from build123d import *

# Parameters (mm, degrees)
SKETCH1_W           = 7.5
SKETCH1_H           = 7.5
BOSS_EXTRUDE1_DEPTH = 40
SKETCH2_W           = 24
SKETCH2_H           = 20
BOSS_EXTRUDE2_DEPTH = 40
SKETCH4_R           = 3.75
CUT_EXTRUDE1_DEPTH  = 20
SKETCH3_R           = 3.25
CUT_EXTRUDE2_DEPTH  = 40


with BuildPart() as part:
    # Sketch1 → Boss-Extrude1 (new body)
    with BuildSketch(Plane(origin=(0, 0, 0), x_dir=(0, 0, -1), z_dir=(1, 0, 0))):
        Rectangle(SKETCH1_W, SKETCH1_H)
    extrude(amount=BOSS_EXTRUDE1_DEPTH)

    # Sketch2 → Boss-Extrude2 (add)
    with BuildSketch(Plane.ZY):
        Rectangle(SKETCH2_W, SKETCH2_H)
    extrude(amount=BOSS_EXTRUDE2_DEPTH)

    # Sketch4 → Cut-Extrude1 (cut)
    with BuildSketch(Plane(origin=(0, 10, 0), x_dir=(1, 0, 0), z_dir=(0, 1, 0))):
        with Locations((-30, 0)):
            Circle(SKETCH4_R)
    extrude(amount=-CUT_EXTRUDE1_DEPTH, mode=Mode.SUBTRACT)

    # Sketch3 → Cut-Extrude2 (cut)
    with BuildSketch(Plane(origin=(40, 0, 0), x_dir=(0, 0, -1), z_dir=(1, 0, 0))):
        Circle(SKETCH3_R)
    extrude(amount=-CUT_EXTRUDE2_DEPTH, mode=Mode.SUBTRACT)


solid = part.part
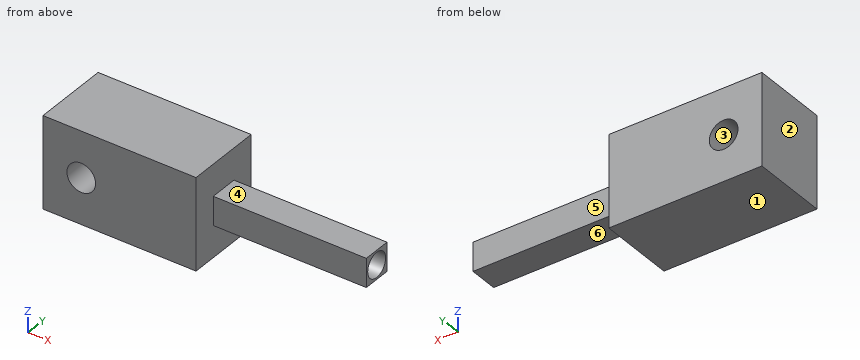
Could you check a few things on this model? Use its own coordinates, in mm. Face numbers are marked on the shaded views. A direction names the side the tool comes from. Round coordinates to 2 decimals unless told otherwise and drop trailing zeros. Write each loop counter-clockwise with the first axis right and the second up, starting at its lowest first coordinate (ties: lowest second). Pieces come first, ordered by that corner, then holes. Notation, with made-up numbers: (65.25, -11) -> (85.25, -11) arc R22 cw to (85.25, 3) -> close; hole circle Ø8 at (-26, 49). An arc over 180 degrees is marked (long way). Use a Markdown table: item, result.
1. We'd pull the mould along Z, two halves only. Please class the marked faces 1, 2 and 3: +Z half, -Z half, draft (parallel to the pull), parting line (faces both ways), or undercut.
Answer key:
| item | result |
|---|---|
| face 1 | -Z half |
| face 2 | draft |
| face 3 | undercut |
2. If we section it at B-B (z = 0): List the corners of the cut face in (x, y) for me.
Answer key:
| item | result |
|---|---|
| outline | (-40, -10) -> (-33.75, -10) -> (-33.75, 10) -> (-40, 10) -> close; (-26.25, -10) -> (0, -10) -> (0, -3.75) -> (40, -3.75) -> (40, -3.25) -> (0, -3.25) -> (0, 3.25) -> (40, 3.25) -> (40, 3.75) -> (0, 3.75) -> (0, 10) -> (-26.25, 10) -> close |
3. Please list where these lines run through material, in increasing order: probe 1 along Y at (x, z) = (14, 0); probe 2 along Z at (x, y) = (-30, 3.75); probe 3 along X at (y, z) = (1, -2.75).
Answer key:
| item | result |
|---|---|
| probe 1 | y = -3.75 to -3.25, 3.25 to 3.75 |
| probe 2 | z = -12 to -3.75, 3.75 to 12 |
| probe 3 | x = -40 to -32.55, -27.45 to 0 |
4. If we section it at C-C (y = 0): List the corners of the cut face in (x, z) for me, then the cut area to 3 significant figures.
Answer key:
| item | result |
|---|---|
| outline | (-40, -12) -> (0, -12) -> (0, -3.75) -> (40, -3.75) -> (40, -3.25) -> (0, -3.25) -> (0, 3.25) -> (40, 3.25) -> (40, 3.75) -> (0, 3.75) -> (0, 12) -> (-40, 12) -> close; hole circle Ø7.5 at (-30, 0) |
| area | 956 mm^2 |
5. If we section it at D-D (x = 17): List the corners of the cut face in (y, z) for me.
Answer key:
| item | result |
|---|---|
| outline | (-3.75, -3.75) -> (3.75, -3.75) -> (3.75, 3.75) -> (-3.75, 3.75) -> close; hole circle Ø6.5 at (0, 0) |
6. If we section it at A-A (x = -27): List the corners of the cut face in (y, z) for me.
Answer key:
| item | result |
|---|---|
| outline | (-10, -12) -> (10, -12) -> (10, -2.25) -> (-10, -2.25) -> close; (-10, 2.25) -> (10, 2.25) -> (10, 12) -> (-10, 12) -> close |
7. For pin 1 Ø4 at (x, z) = (15.5, -1.5) entering from -Y; pin 2 Ø2 at (x, y) = (21, 0.5) entering from -Z; pin 3 Ø2 at (x, y) = (15, 2) entering from +Z; pin 4 Ø10 at (y, z) = (-5, 3.5) entering from +X, each with a flat end and sliding along its axis, tell me the tip position at first contact or that it passes through.
Answer key:
| item | result |
|---|---|
| pin 1 | stops at y = -3.75 |
| pin 2 | stops at z = -3.75 |
| pin 3 | stops at z = 3.75 |
| pin 4 | stops at x = 40 |
8. Which directions (+Z, -Z, +X, -X, +Y, -Y) give clear straight access to the entire face, cutting with the end or side of a thin tool? Please do the marked faces 4, 5 and 6.
Answer key:
| item | result |
|---|---|
| face 4 | +Z, +X, +Y, -Y |
| face 5 | +Z, -Z, +X, +Y |
| face 6 | -Z, +X, +Y, -Y |
